The listing builds one solid part. Answer for the finished solid, in the listing's coordinates (mm). A direction names the side the tool comes from. Give positions to 0.01 mm unless a question says otherwise; leave off trailing zeros. Loops run counter-clockwise (first coordinate to the right, second up) from the corner with the lowest first, then second, coordinate; pieces in that order, holes last. Notation, with made-up numbers: (84.25, 17.5) - (112.25, 17.5) arc R14 cw to (112.25, 38.5) - close; hole circle Ø1 at (35, 18). An arc over 180 degrees is marked (long way). Answer as CSV lines item,"result". Start each with the question number.
1) Find the intervals of material crossed by line 1 along Z through (x, y) = (15.5, 37); line 2 along X through (y, z) = (19.5, 2); line 3 along Z through (x, y) = (5.5, 60.5), in increasing order.
2) A cutting plane is placed at C-C (z = -5.5). Determine the outline of the cut face in (x, y), and give its area (3 significant figures).
3) A cutting plane is placed at A-A (y = 81). Determine the outline of the cut face in (x, z).
4) For faces 1 (the face through (9, 0, -1)), 2 (the face through (13, 79, 1)), 3 (the face through (4, 79, 0)), determine the directions among +Z, -Z, +X, -X, +Y, -Y from which every point of the face is accessible in a straight line to the end or side of a thin tool.
5) A cutting plane is placed at B-B (x = 3.5). Determine the outline of the cut face in (y, z).
6) Flat-ended cylindrical pins translate along their axes: pin 1 (1.5 mm diameter, centred on y = 16.5, z = -4, fed in from -X); pin 2 (1.5 mm diameter, centred on x = 2, z = -1.5, fed in from +Y); pin 3 (5 mm diameter, centred on x = 13.5, y = 79, fed in from +Z); pin 4 (5.5 mm diameter, centred on y = 120, z = 1, fed in from +X). Find the tip coordinate at first contact, or state that the pin passes through.
```python
from build123d import *

# Parameters (mm, degrees)
BOSS_EXTRUDE1_DEPTH = 160
SKETCH2_W           = 5
SKETCH2_H           = 160
BOSS_EXTRUDE2_DEPTH = 5


with BuildPart() as part:
    # Sketch1 → Boss-Extrude1 (new body)
    with BuildSketch(Plane(origin=(0, 0, 0), x_dir=(1, 0, 0), z_dir=(0, 1, 0))):
        Polygon((0, 0), (8, 0), (8, 7), (13, 7), (13, -5), (8, -5), (0, -5), align=None)
    extrude(amount=BOSS_EXTRUDE1_DEPTH)

    # Sketch2 → Boss-Extrude2 (add)
    with BuildSketch(Plane(origin=(13, 0, 0), x_dir=(0, 0, -1), z_dir=(1, 0, 0))):
        with Locations((4.5, 80)):
            Rectangle(SKETCH2_W, SKETCH2_H)
    extrude(amount=BOSS_EXTRUDE2_DEPTH)


solid = part.part
```
Ans:
1,line 1,"-7 to -2"
1,line 2,"0 to 13"
1,line 3,"0 to 5"
2,outline,"(8, 0) - (18, 0) - (18, 160) - (8, 160) - close"
2,area,"1,600 mm2"
3,outline,"(0, 0) - (8, 0) - (8, -7) - (18, -7) - (18, -2) - (13, -2) - (13, 5) - (0, 5) - close"
4,face 1,"+Z, -Z, +X, -X, -Y"
4,face 2,"+Z, +X, +Y, -Y"
4,face 3,"-Z, -X, +Y, -Y"
5,outline,"(0, 0) - (160, 0) - (160, 5) - (0, 5) - close"
6,pin 1,"x = 8"
6,pin 2,"through"
6,pin 3,"z = 5"
6,pin 4,"x = 13"
